Geometry: final body of the model. Coordinates: model frame, mm. A direction names the side the tool comes from. Give positions to 0.01 mm unless a question says otherwise; leave off trailing zeros.
Q1. Pin query (flat end, axial travel): pin 1 Ø7 at (y, z) = (-522, -93.5) entering from -X; pin 2 Ø4 at (x, y) = (1, -207.5) entering from +Z; pin 3 Ø3 at (x, y) = (2, -243) entering from -Z. Return the tip coordinate at first contact, or that it passes through.
Q2. Reachability of faces 3 (the flat face through (-4, -351, 100)), 4 (the flat face through (0, 0, 1)), 5 (the flat face through (7, -351, -35)) from +Z, -Z, +X, -X, +Y, -Y: full face, straight path, thin tool, end or side. Return the list, or none.
Q3. Line query: line 1 (X direction, y = -117, z = 63); line 2 (X direction, y = -424, z = -7); line 3 (Z direction, x = -10, y = -174). Output: solid intervals per line, ascending.
Q4. Section A-A (y = -624). State how many separate pieces and enclosed holes the cut face has, plus the area to 3 significant figures.
Q5. Mould query, pull axis Z, two halves, no side actions, for faces 1 (the flat face through (7, -351, -61)), 2 (the flat face through (-15, -351, 22)). Classes: +Z half, -Z half, draft (parallel to the pull), parting line (faces both ways), or undercut.
from build123d import *

# Parameters (mm, degrees)
F1_DEPTH = 711.2
F3_DEPTH = 711.2


# Not quite as in the source:
# - ends of sketch curves that miss each other by under 0.0002 mm in the source are joined


with BuildPart() as f1:
    # F0 (on Front) → F1 (new body)
    with BuildSketch(Plane.XZ):
        with BuildLine():
            ThreePointArc((-14.9999680608, -58.9985104), (-14.96444377, -59.322873513), (-14.8595551032, -59.6318585804))
            Line((-14.8595551032, -59.6318585804), (-11.0988328608, -67.6967912))
            ThreePointArc((-11.0988328608, -67.6967912), (-11.1617050028, -68.655791158), (-12.004294, -69.1180454046))
            Line((-12.004294, -69.1180454046), (-14.0009118, -69.1180736))
            ThreePointArc((-14.0009118, -69.1180736), (-14.707352628, -69.410690972), (-14.99997, -70.1171318))
            Line((-14.99997, -70.1171318), (-14.99997, -85.599397))
            ThreePointArc((-14.99997, -85.599397), (-14.5606310505, -86.6600550505), (-13.499973, -87.099394))
            Line((-13.499973, -87.099394), (-5.5003446, -87.099394))
            ThreePointArc((-5.5003446, -87.099394), (-4.4396865495, -86.6600550505), (-4.0003476, -85.599397))
            Line((-4.0003476, -85.599397), (-4.0003476, -80.5996356))
            ThreePointArc((-4.0003476, -80.5996356), (-3.5610086505, -79.5389775495), (-2.5003506, -79.0996386))
            Line((-2.5003506, -79.0996386), (1.4838426, -79.0996386))
            ThreePointArc((1.4838426, -79.0996386), (2.5445365709, -79.5390134712), (2.9838395966, -80.5997372))
            Line((2.9838395966, -80.5997372), (2.98196, -104.5986224))
            ThreePointArc((2.98196, -104.5986224), (3.4212540492, -105.6593625482), (4.481957, -106.0987464))
            Line((4.481957, -106.0987464), (13.499973, -106.0987464))
            ThreePointArc((13.499973, -106.0987464), (14.5606310505, -105.6594074505), (14.99997, -104.5987494))
            Line((14.99997, -104.5987494), (14.99997, 83.7761342))
            ThreePointArc((14.99997, 83.7761342), (14.5844487053, 84.8124273268), (13.5680958768, 85.2745834897))
            Line((13.5680958768, 85.2745834897), (5.104384, 85.6592902))
            ThreePointArc((5.104384, 85.6592902), (4.5671403109, 85.7853117853), (4.1118233495, 86.0970797495))
            Line((4.1118233495, 86.0970797495), (-3.5610038, 93.7699166))
            ThreePointArc((-3.5610038, 93.7699166), (-3.8861671271, 94.2565457995), (-4.0003476, 94.8305698))
            Line((-4.0003476, 94.8305698), (-4.0003476, 106.0987464))
            Line((-4.0003476, 106.0987464), (-12.3105164, 106.0987464))
            Line((-12.3105164, 106.0987464), (-14.99997, 101.2086876))
            Line((-14.99997, 101.2086876), (-14.9999680608, -58.9985104))
        make_face()
    extrude(amount=F1_DEPTH)

    # F2 (on Front) → F3 (cut)
    with BuildSketch(Plane.XZ):
        with BuildLine():
            ThreePointArc((-5.49529, -31.195264), (-4.4346319495, -31.6346029495), (-3.995293, -32.695261))
            Line((-3.995293, -32.695261), (-3.995293, -37.695251))
            ThreePointArc((-3.995293, -37.695251), (-4.4346319495, -38.7559090505), (-5.49529, -39.195248))
            Line((-5.49529, -39.195248), (-5.499989, -39.195248))
            ThreePointArc((-5.499989, -39.195248), (-6.5606470505, -39.6345869495), (-6.999986, -40.695245))
            Line((-6.999986, -40.695245), (-6.999986, -41.195244))
            ThreePointArc((-6.999986, -41.195244), (-6.1213081009, -43.3165601009), (-3.999992, -44.195238))
            Line((-3.999992, -44.195238), (3.999992, -44.195238))
            ThreePointArc((3.999992, -44.195238), (6.1213081009, -43.3165601009), (6.999986, -41.195244))
            Line((6.999986, -41.195244), (6.999986, -29.195268))
            ThreePointArc((6.999986, -29.195268), (6.1213081009, -27.0739518991), (3.999992, -26.195274))
            Line((3.999992, -26.195274), (-3.999992, -26.195274))
            ThreePointArc((-3.999992, -26.195274), (-6.1213081009, -27.0739518991), (-6.999986, -29.195268))
            Line((-6.999986, -29.195268), (-6.999986, -29.695267))
            ThreePointArc((-6.999986, -29.695267), (-6.5606470505, -30.7559250505), (-5.499989, -31.195264))
            Line((-5.499989, -31.195264), (-5.49529, -31.195264))
        make_face()
        with BuildLine():
            ThreePointArc((-5.49529, -56.595264), (-4.4346319495, -57.0346029495), (-3.995293, -58.095261))
            Line((-3.995293, -58.095261), (-3.995293, -63.095251))
            ThreePointArc((-3.995293, -63.095251), (-4.4346319495, -64.1559090505), (-5.49529, -64.595248))
            Line((-5.49529, -64.595248), (-5.499989, -64.595248))
            ThreePointArc((-5.499989, -64.595248), (-6.5606470505, -65.0345869495), (-6.999986, -66.095245))
            Line((-6.999986, -66.095245), (-6.999986, -66.595244))
            ThreePointArc((-6.999986, -66.595244), (-6.1213081009, -68.7165601009), (-3.999992, -69.595238))
            Line((-3.999992, -69.595238), (0, -69.595238))
            Line((0, -69.595238), (3.999992, -69.595238))
            ThreePointArc((3.999992, -69.595238), (6.1213081009, -68.7165601009), (6.999986, -66.595244))
            Line((6.999986, -66.595244), (6.999986, -54.595268))
            ThreePointArc((6.999986, -54.595268), (6.1213081009, -52.4739518991), (3.999992, -51.595274))
            Line((3.999992, -51.595274), (-3.999992, -51.595274))
            ThreePointArc((-3.999992, -51.595274), (-6.1213081009, -52.4739518991), (-6.999986, -54.595268))
            Line((-6.999986, -54.595268), (-6.999986, -55.095267))
            ThreePointArc((-6.999986, -55.095267), (-6.5606470505, -56.1559250505), (-5.499989, -56.595264))
            Line((-5.499989, -56.595264), (-5.49529, -56.595264))
        make_face()
        with BuildLine():
            ThreePointArc((-5.49529, -5.3953664), (-4.4346319495, -5.8347053495), (-3.995293, -6.8953634))
            Line((-3.995293, -6.8953634), (-3.995293, -11.8953534))
            ThreePointArc((-3.995293, -11.8953534), (-4.4346319495, -12.9560114505), (-5.49529, -13.3953504))
            Line((-5.49529, -13.3953504), (-5.499989, -13.3953504))
            ThreePointArc((-5.499989, -13.3953504), (-6.5606470505, -13.8346893495), (-6.999986, -14.8953474))
            Line((-6.999986, -14.8953474), (-6.999986, -15.3953464))
            ThreePointArc((-6.999986, -15.3953464), (-6.1213081009, -17.5166625009), (-3.999992, -18.3953404))
            Line((-3.999992, -18.3953404), (3.999992, -18.3953404))
            ThreePointArc((3.999992, -18.3953404), (6.1213081009, -17.5166625009), (6.999986, -15.3953464))
            Line((6.999986, -15.3953464), (6.999986, -3.3953704))
            ThreePointArc((6.999986, -3.3953704), (6.1213081009, -1.2740542991), (3.999992, -0.3953764))
            Line((3.999992, -0.3953764), (-3.999992, -0.3953764))
            ThreePointArc((-3.999992, -0.3953764), (-6.1213081009, -1.2740542991), (-6.999986, -3.3953704))
            Line((-6.999986, -3.3953704), (-6.999986, -3.8953694))
            ThreePointArc((-6.999986, -3.8953694), (-6.5606470505, -4.9560274505), (-5.499989, -5.3953664))
            Line((-5.499989, -5.3953664), (-5.49529, -5.3953664))
        make_face()
        with BuildLine():
            Line((-5.499989, 20.4015086), (-5.49529, 20.4015086))
            ThreePointArc((-5.49529, 20.4015086), (-4.4346319495, 19.9621696505), (-3.995293, 18.9015116))
            Line((-3.995293, 18.9015116), (-3.995293, 13.9015216))
            ThreePointArc((-3.995293, 13.9015216), (-4.4346319495, 12.8408635495), (-5.49529, 12.4015246))
            Line((-5.49529, 12.4015246), (-5.499989, 12.4015246))
            ThreePointArc((-5.499989, 12.4015246), (-6.5606470505, 11.9621856505), (-6.999986, 10.9015276))
            Line((-6.999986, 10.9015276), (-6.999986, 10.4015286))
            ThreePointArc((-6.999986, 10.4015286), (-6.1213081009, 8.2802124991), (-3.999992, 7.4015346))
            Line((-3.999992, 7.4015346), (3.999992, 7.4015346))
            ThreePointArc((3.999992, 7.4015346), (6.1213081009, 8.2802124991), (6.999986, 10.4015286))
            Line((6.999986, 10.4015286), (6.999986, 22.4015046))
            ThreePointArc((6.999986, 22.4015046), (6.1213081009, 24.5228207009), (3.999992, 25.4014986))
            Line((3.999992, 25.4014986), (-3.999992, 25.4014986))
            ThreePointArc((-3.999992, 25.4014986), (-6.1213081009, 24.5228207009), (-6.999986, 22.4015046))
            Line((-6.999986, 22.4015046), (-6.999986, 21.9015056))
            ThreePointArc((-6.999986, 21.9015056), (-6.5606470505, 20.8408475495), (-5.499989, 20.4015086))
        make_face()
        with BuildLine():
            Line((-5.499989, 46.1983836), (-5.49529, 46.1983836))
            ThreePointArc((-5.49529, 46.1983836), (-4.4346319495, 45.7590446505), (-3.995293, 44.6983866))
            Line((-3.995293, 44.6983866), (-3.995293, 39.6983966))
            ThreePointArc((-3.995293, 39.6983966), (-4.4346319495, 38.6377385495), (-5.49529, 38.1983996))
            Line((-5.49529, 38.1983996), (-5.499989, 38.1983996))
            ThreePointArc((-5.499989, 38.1983996), (-6.5606470505, 37.7590606505), (-6.999986, 36.6984026))
            Line((-6.999986, 36.6984026), (-6.999986, 36.1984036))
            ThreePointArc((-6.999986, 36.1984036), (-6.1213081009, 34.0770874991), (-3.999992, 33.1984096))
            Line((-3.999992, 33.1984096), (3.999992, 33.1984096))
            ThreePointArc((3.999992, 33.1984096), (6.1213081009, 34.0770874991), (6.999986, 36.1984036))
            Line((6.999986, 36.1984036), (6.999986, 48.1983796))
            ThreePointArc((6.999986, 48.1983796), (6.1213081009, 50.3196957009), (3.999992, 51.1983736))
            Line((3.999992, 51.1983736), (-3.999992, 51.1983736))
            ThreePointArc((-3.999992, 51.1983736), (-6.1213081009, 50.3196957009), (-6.999986, 48.1983796))
            Line((-6.999986, 48.1983796), (-6.999986, 47.6983806))
            ThreePointArc((-6.999986, 47.6983806), (-6.5606470505, 46.6377225495), (-5.499989, 46.1983836))
        make_face()
        with BuildLine():
            Line((-5.499989, 71.9952586), (-5.49529, 71.9952586))
            ThreePointArc((-5.49529, 71.9952586), (-4.4346319495, 71.5559196505), (-3.995293, 70.4952616))
            Line((-3.995293, 70.4952616), (-3.995293, 65.4952716))
            ThreePointArc((-3.995293, 65.4952716), (-4.4346319495, 64.4346135495), (-5.49529, 63.9952746))
            Line((-5.49529, 63.9952746), (-5.499989, 63.9952746))
            ThreePointArc((-5.499989, 63.9952746), (-6.5606470505, 63.5559356505), (-6.999986, 62.4952776))
            Line((-6.999986, 62.4952776), (-6.999986, 61.9952786))
            ThreePointArc((-6.999986, 61.9952786), (-6.1213081009, 59.8739624991), (-3.999992, 58.9952846))
            Line((-3.999992, 58.9952846), (3.999992, 58.9952846))
            ThreePointArc((3.999992, 58.9952846), (6.1213081009, 59.8739624991), (6.999986, 61.9952786))
            Line((6.999986, 61.9952786), (6.999986, 73.9952546))
            ThreePointArc((6.999986, 73.9952546), (6.1213081009, 76.1165707009), (3.999992, 76.9952486))
            Line((3.999992, 76.9952486), (-3.999992, 76.9952486))
            ThreePointArc((-3.999992, 76.9952486), (-6.1213081009, 76.1165707009), (-6.999986, 73.9952546))
            Line((-6.999986, 73.9952546), (-6.999986, 73.4952556))
            ThreePointArc((-6.999986, 73.4952556), (-6.5606470505, 72.4345975495), (-5.499989, 71.9952586))
        make_face()
    extrude(amount=F3_DEPTH, mode=Mode.SUBTRACT)


solid = f1.part
Computed:
1. pin 1: stops at x = 2.98
1. pin 2: stops at z = 91.21
1. pin 3: stops at z = -105.73
2. face 3: +Z, +X, +Y, -Y
2. face 4: +Z, -Z, +X, -X, +Y
2. face 5: +Y, -Y
3. line 1: x = -15 to -6.91, 7 to 15
3. line 2: x = -15 to -4, 7 to 15
3. line 3: z = -87.1 to 106.1
4. separate pieces: 1
4. enclosed holes: 6
4. area: 4,260 mm2
5. face 1: undercut
5. face 2: draft
